from build123d import *

# Parameters (mm, degrees)
PAD_DEPTH             = 4
POCKET_DEPTH          = 129.213319
POLARPATTERN_COUNT    = 8
POLARPATTERN_ANGLE    = 135
POCKET001_DEPTH       = 163.025541
POLARPATTERN001_COUNT = 8
POLARPATTERN001_ANGLE = 135
FILLET_R              = 4
CHAMFER_SIZE          = 1
CHAMFER001_SIZE       = 1
SKETCH004_W           = 2
SKETCH004_H           = 2
POCKET002_DEPTH       = 4.001


with BuildPart() as part:
    # Sketch → Pad (new body)
    with BuildSketch(Plane.XY):
        with BuildLine():
            ThreePointArc((5.7, -22.076005), (22.618277, 2.872898), (0, 22.8))
            Line((0, 22.8), (0, 28.3))
            ThreePointArc((7.075, -27.401357), (28.07444, 3.565921), (0, 28.3))
            Line((5.7, -22.076005), (7.075, -27.401357))
        make_face()
    pad = extrude(amount=PAD_DEPTH)

    # Sketch001 → Pocket (cut, through all)
    with BuildSketch(Plane.XY):
        with BuildLine():
            Line((0, 0), (10.448469, -20.264982))
            ThreePointArc((10.448469, -20.264982), (12.887389, -22.743593), (12.014528, -19.377593))
            Line((12.014528, -19.377593), (0, 0))
        make_face()
    pocket = extrude(amount=POCKET_DEPTH, mode=Mode.SUBTRACT)

    # PolarPattern: Pocket ×8 about axis
    polarpattern_axis = Axis((0, 0, 0), (0, 0, 1))
    for i in range(1, POLARPATTERN_COUNT):
        add(pocket.rotate(polarpattern_axis, i * POLARPATTERN_ANGLE / (POLARPATTERN_COUNT - 1)), mode=Mode.SUBTRACT)

    # Mirrored: Pad across Sketch V_Axis
    add(pad.mirror(Plane(origin=(0, 0, 0), x_dir=(0, 0, 1), z_dir=(1, 0, 0))))

    # Sketch003 → Pocket001 (cut, through all)
    with BuildSketch(Plane.XY):
        with BuildLine():
            Line((0, 0), (-12.014528, -19.377593))
            ThreePointArc((-12.014528, -19.377593), (-12.887389, -22.743593), (-10.448469, -20.264982))
            Line((-10.448469, -20.264982), (0, 0))
        make_face()
    pocket001 = extrude(amount=POCKET001_DEPTH, mode=Mode.SUBTRACT)

    # PolarPattern001: Pocket001 ×8 about axis
    polarpattern001_axis = Axis((0, 0, 0), (0, 0, -1))
    for i in range(1, POLARPATTERN001_COUNT):
        add(pocket001.rotate(polarpattern001_axis, i * POLARPATTERN001_ANGLE / (POLARPATTERN001_COUNT - 1)), mode=Mode.SUBTRACT)

    # Fillet
    fillet_edges = [part.edges().sort_by_distance(p)[0] for p in [
        (7.075, -27.401357, 2),
        (-7.075, -27.401357, 2),
    ]]
    fillet(fillet_edges, radius=FILLET_R)

    # Chamfer
    chamfer_edges = [part.edges().sort_by_distance(p)[0] for p in [
        (8.125118, -25.809145, 4),
        (27.684037, 5.872314, 4),
        (-27.684037, 5.872314, 4),
        (-8.125118, -25.809145, 4),
        (-5.846065, -22.641713, 4),
        (5.846065, -22.641713, 4),
    ]]
    chamfer(chamfer_edges, length=CHAMFER_SIZE)

    # Chamfer001
    chamfer001_edges = [part.edges().sort_by_distance(p)[0] for p in [
        (-8.125118, -25.809145, 0),
        (-5.846065, -22.641713, 0),
        (-27.684037, 5.872314, 0),
        (27.684037, 5.872314, 0),
        (8.125118, -25.809145, 0),
        (5.846065, -22.641713, 0),
    ]]
    chamfer(chamfer001_edges, length=CHAMFER001_SIZE)

    # Sketch004 → Pocket002 (cut, through all)
    with BuildSketch(Plane.XY):
        with Locations((0, 25.25)):
            Rectangle(SKETCH004_W, SKETCH004_H)
    extrude(amount=POCKET002_DEPTH, mode=Mode.SUBTRACT)


solid = part.part
Could you check a few things on this model? Use its own coordinates, in mm. A direction names the side the tool comes from. Coordinates: 2 decimals unless noted, no trailing zeros.
1. I need wall thicknesses on L1, parallel to Y at x = 24.5, z = 0.8; L2, parallel to Y at x = 13.5, z = 3.25; L3, parallel to X at y = 22, z = 2.5. Which ranges of each line are inside material? Lowest first, please.
2. For faces 3 (the face through (6.34, -22.51, 0.49)), 4 (the face through (0, 24.25, 2)), which set-ups out of +Z, -Z, +X, -X, +Y, -Y let a thin tool reach every point of the face, with its end or its side?
3. We'd pull the mould along Y, two halves only. Please class faces 1 (the face through (6.34, -22.51, 3.51)), 2 (the face through (19.63, -17.26, 1.97)): released by +Y, released by -Y, zero draft, split by the parting line, or undercut.
4. For P1, Ø1, axis at x = 0, z = 2.5, coming from the -Y side; P2, Ø1.5, axis at x = 9, z = 2.5, coming from the +Y side; P3, Ø1.5, axis at x = 2, z = 3.5, coming from the +Y side, each with a flat end and sliding along its axis, tell me the tip position at first contact or that it passes through.
Computed values:
1. L1: y = -13.76 to -2.9, 0.68 to 5.63, 8.34 to 13.76
1. L2: y = -24.59 to -22.17, -20.18 to -18.37, 21.76 to 24.59
1. L3: x = -17.8 to -7.54, 7.54 to 17.8
2. face 3: -Z, -Y
2. face 4: +Z, -Z
3. face 1: released by -Y
3. face 2: undercut
4. P1: stops at y = 22.79
4. P2: stops at y = 27.07
4. P3: stops at y = 28.26
